Can you work these out from the model? Positions are in its coordinate system, mm. A direction names the side the tool comes from. Give positions to 0.01 mm unless a question says otherwise; leave off trailing zeros. Loops run counter-clockwise (first coordinate to the right, second up) from the corner with the lowest first, then second, coordinate; pieces in that order, holes last. Notation, with made-up numbers: M 38,43.25 L 44,43.25 A21 cw 44,76.25 Z; hole C 71,-15 d11. An arc over 180 degrees is marked long. Put each result on its own line as item: value. Start each with the question number.
1) Imagine slicing it at C-C (x = 9.5). Write out the boundary of the cut face in (y, z).
2) If we mould it in two halves opening along Y, with no side actions, what happens to faces 1 (the flat face through (20, 40.457, 25)), 2 (the cylindrical face through (1.33, 38.17, 24.65)), 3 (the flat face through (13, 26, 50))? For each: +Y half, -Y half, draft (parallel to the pull), parting line (faces both ways), or undercut.
3) Imagine slicing it at B-B (y = 3.5). Write out the boundary of the cut face in (x, z), then the cut area to 3 significant figures.
4) For P1, Ø2, axis at x = -25, z = 7, coming from the -Y side; P2, Ø10, axis at x = 1.5, z = 30, coming from the -Y side; P3, Ø1, axis at y = 18.5, z = 26.5, coming from the -X side; P4, Ø3, axis at x = 9.5, y = 2, coming from the +Z side, each with a flat end and sliding along its axis, tell me the tip position at first contact or that it passes through.
5) Imagine slicing it at D-D (x = 1). Write out the boundary of the cut face in (y, z).
6) Please list where these lines run through material, in increasing order: line 1 along Y through (x, z) = (40.5, 14.5); line 2 along Y through (x, z) = (5.5, 27); line 3 along Y through (x, z) = (5, 44). Write a range as from..to.
7) For faces 4 (the flat face through (27, 35.457, 25)), 5 (the flat face through (13, 26, 0)), which set-ups out of +Z, -Z, +X, -X, +Y, -Y let a thin tool reach every point of the face, with its end or its side?
8) Imagine slicing it at A-A (x = 30.5). Write out the boundary of the cut face in (y, z), then the cut area to 3 significant figures.
from build123d import *

# Parameters (mm, degrees)
F1_DEPTH = 50
F3_D     = 50


# Not quite as in the source:
# - the program builds the solid bodies; features that only make, move or delete a surface that nothing else refers to are left out


with BuildPart() as f1:
    # F0 (on Top) → F1 (new body)
    with BuildSketch(Plane.XY):
        with BuildLine():
            Line((49.3272994906, 40.4565469784), (-10.1727005094, 40.4565469784))
            ThreePointArc((-10.1727005094, 40.4565469784), (-17.0425953064, -10.3691748199), (5.9889720653, 35.4565423621))
            Line((5.9889720653, 35.4565423621), (49.2908384362, 35.4565423621))
            Line((49.2908384362, 35.4565423621), (49.2908384362, 36.4565423621))
            Line((49.2908384362, 36.4565423621), (4.5184440125, 36.4565423621))
            ThreePointArc((4.5184440125, 36.4565423621), (1.2797957907, 38.1934060872), (-2.1713849513, 39.4562953896))
            Line((-2.1713849513, 39.4562953896), (49.3272994906, 39.4562953896))
            Line((49.3272994906, 39.4562953896), (49.3272994906, 40.4565469784))
        make_face()
        with BuildLine():
            ThreePointArc((-10.1647124973, 39.4562953896), (8.0319806239, 32.4298558016), (15.6417905006, 14.4693077177))
            ThreePointArc((15.6417905006, 14.4693077177), (-26.7483996228, -3.4912403662), (-10.1647124973, 39.4562953896))
        make_face(mode=Mode.SUBTRACT)
        with BuildLine():
            ThreePointArc((-10.1647124973, 39.4562953896), (-26.7483996228, -3.4912403662), (15.6417905006, 14.4693077177))
            ThreePointArc((15.6417905006, 14.4693077177), (8.0319806239, 32.4298558016), (-10.1647124973, 39.4562953896))
        make_face()
    extrude(amount=F1_DEPTH)

    # F3 (through all)
    with Locations(Plane(origin=(0, 0, 0), x_dir=(1, 0, 0), z_dir=(0, 0, -1))):
        with Locations((-9.3582094994, -14.4693077177)):
            Hole(F3_D / 2)


solid = f1.part
Recorded:
1. outline: M -3.43,0 L -1.94,0 L -1.94,50 L -3.43,50 Z; M 30.88,0 L 32.37,0 L 32.37,50 L 30.88,50 Z; M 35.46,0 L 36.46,0 L 36.46,50 L 35.46,50 Z; M 39.46,0 L 40.46,0 L 40.46,50 L 39.46,50 Z
2. face 1: +Y half
2. face 2: undercut
2. face 3: draft
3. outline: M -32.93,0 L -31.82,0 L -31.82,50 L -32.93,50 Z; M 13.11,0 L 14.21,0 L 14.21,50 L 13.11,50 Z
3. area: 111 mm²
4. P1: y = -7.02
4. P2: y = -10.86
4. P3: x = -35.12
4. P4: through
5. outline: M -9.38,0 L -8.28,0 L -8.28,50 L -9.38,50 Z; M 37.22,0 L 38.32,0 L 38.32,50 L 37.22,50 Z; M 39.46,0 L 40.46,0 L 40.46,50 L 39.46,50 Z
6. line 1: 35.46..36.46, 39.46..40.46
6. line 2: -6.87..-5.64, 34.57..36.46, 39.46..40.46
6. line 3: -7.21..-6, 34.93..36.46, 39.46..40.46
7. face 4: +Z, -Z, +X
7. face 5: -Z, +X, -X, +Y, -Y
8. outline: M 35.46,0 L 36.46,0 L 36.46,50 L 35.46,50 Z; M 39.46,0 L 40.46,0 L 40.46,50 L 39.46,50 Z
8. area: 100 mm²
